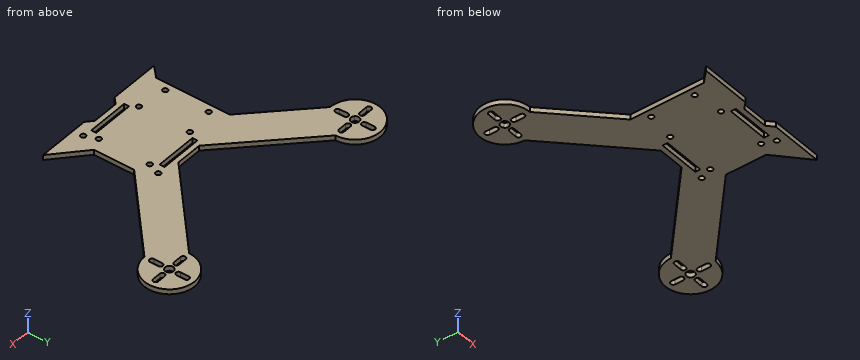
```python
from build123d import *

# Parameters (mm, degrees)
F0_R     = 1.5
F0_W     = 25
F0_H     = 3
F0_R_2   = 2.5
F1_DEPTH = 3


# Not quite as in the source:
# - ends of sketch curves that miss each other by under 0.0002 mm in the source are joined


with BuildPart() as f1:
    # F0 (on Top) → F1 (new body)
    with BuildSketch(Plane.XY):
        with BuildLine():
            Line((-10.0000000587, 25), (-55.7106781187, 70.7106779065))
            ThreePointArc((-55.7106781187, 70.7106779065), (-81.3172799026, 81.3172797703), (-70.7106779065, 55.7106781187))
            Line((-70.7106779065, 55.7106781187), (-37, 22.0000003253))
            Line((-37, 22.0000003253), (-37, -22.0000003253))
            Line((-37, -22.0000003253), (-43.4767450368, -28.4767453404))
            Line((-43.4767450368, -28.4767453404), (-13.4767454108, -28.4767453404))
            Line((-13.4767454108, -28.4767453404), (-10.0000000587, -25))
            Line((-10.0000000587, -25), (5.8262266936, -25))
            Line((5.8262266936, -25), (9.6204284269, -28.4767453404))
            Line((9.6204284269, -28.4767453404), (40.9900556349, -28.4767453404))
            Line((40.9900556349, -28.4767453404), (23, -11.9918965954))
            Line((23, -11.9918965954), (23, 11.9918965954))
            Line((23, 11.9918965954), (70.7106780935, 55.7106781187))
            ThreePointArc((70.7106780935, 55.7106781187), (81.3172798365, 81.3172798365), (55.7106781187, 70.7106779065))
            Line((55.7106781187, 70.7106779065), (5.8262266936, 25))
            Line((5.8262266936, 25), (-10.0000000587, 25))
        make_face()
        with Locations((-15.25, -15.25)):
            Circle(F0_R, mode=Mode.SUBTRACT)
        with Locations((-32.5, -13)):
            Circle(F0_R, mode=Mode.SUBTRACT)
        with Locations((-32.5, 13)):
            Circle(F0_R, mode=Mode.SUBTRACT)
        with Locations((-15.25, 15.25)):
            Circle(F0_R, mode=Mode.SUBTRACT)
        with Locations((18, -22.5)):
            Circle(F0_R, mode=Mode.SUBTRACT)
        with Locations((0, -20.5)):
            Rectangle(F0_W, F0_H, mode=Mode.SUBTRACT)
        with Locations((15.25, -15.25)):
            Circle(F0_R, mode=Mode.SUBTRACT)
        with Locations((0, 20.5)):
            Rectangle(F0_W, F0_H, mode=Mode.SUBTRACT)
        with Locations((15.25, 15.25)):
            Circle(F0_R, mode=Mode.SUBTRACT)
        with Locations((18, 22.5)):
            Circle(F0_R, mode=Mode.SUBTRACT)
        with BuildLine():
            ThreePointArc((-72.2106780183, 65.2703154499), (-70.7106780132, 66.7703154448), (-69.2106780183, 65.2703154398))
            Line((-69.2106780183, 65.2703154398), (-69.210678035, 60.2703154398))
            ThreePointArc((-69.210678035, 60.2703154398), (-70.7106780401, 58.7703154448), (-72.210678035, 60.2703154499))
            Line((-72.210678035, 60.2703154499), (-72.2106780183, 65.2703154499))
        make_face(mode=Mode.SUBTRACT)
        with BuildLine():
            ThreePointArc((-76.1510407975, 72.2106782191), (-74.6510407925, 70.7106782241), (-76.1510407874, 69.2106782191))
            Line((-76.1510407874, 69.2106782191), (-81.1510407874, 69.2106782023))
            ThreePointArc((-81.1510407874, 69.2106782023), (-82.6510407925, 70.7106781972), (-81.1510407975, 72.2106782023))
            Line((-81.1510407975, 72.2106782023), (-76.1510407975, 72.2106782191))
        make_face(mode=Mode.SUBTRACT)
        with BuildLine():
            ThreePointArc((-68.9429111657, 72.4784450716), (-68.4009792874, 71.6673866996), (-68.2106781187, 70.7106781187))
            ThreePointArc((-68.2106781187, 70.7106781187), (-69.7539695377, 68.4009792874), (-72.4784450716, 68.9429111657))
            ThreePointArc((-72.4784450716, 68.9429111657), (-72.4784450716, 72.4784450716), (-68.9429111657, 72.4784450716))
        make_face(mode=Mode.SUBTRACT)
        with BuildLine():
            Line((-60.2703154398, 69.210678035), (-65.2703154398, 69.2106780183))
            ThreePointArc((-65.2703154398, 69.2106780183), (-66.7703154448, 70.7106780132), (-65.2703154499, 72.2106780183))
            Line((-65.2703154499, 72.2106780183), (-60.2703154499, 72.210678035))
            ThreePointArc((-60.2703154499, 72.210678035), (-58.7703154448, 70.7106780401), (-60.2703154398, 69.210678035))
        make_face(mode=Mode.SUBTRACT)
        with BuildLine():
            Line((-69.210678, 81.1510407925), (-69.210678, 76.1510407925))
            ThreePointArc((-69.210678, 76.1510407925), (-70.710678, 74.6510407925), (-72.210678, 76.1510407925))
            Line((-72.210678, 76.1510407925), (-72.210678, 81.1510407925))
            ThreePointArc((-72.210678, 81.1510407925), (-70.710678, 82.6510407925), (-69.210678, 81.1510407925))
        make_face(mode=Mode.SUBTRACT)
        with BuildLine():
            ThreePointArc((65.2703154499, 72.2106780183), (66.7703154448, 70.7106780132), (65.2703154398, 69.2106780183))
            Line((65.2703154398, 69.2106780183), (60.2703154398, 69.210678035))
            ThreePointArc((60.2703154398, 69.210678035), (58.7703154448, 70.7106780401), (60.2703154499, 72.210678035))
            Line((60.2703154499, 72.210678035), (65.2703154499, 72.2106780183))
        make_face(mode=Mode.SUBTRACT)
        with BuildLine():
            Line((69.210678035, 60.2703154398), (69.2106780183, 65.2703154398))
            ThreePointArc((69.2106780183, 65.2703154398), (70.7106780132, 66.7703154448), (72.2106780183, 65.2703154499))
            Line((72.2106780183, 65.2703154499), (72.210678035, 60.2703154499))
            ThreePointArc((72.210678035, 60.2703154499), (70.7106780401, 58.7703154448), (69.210678035, 60.2703154398))
        make_face(mode=Mode.SUBTRACT)
        with Locations((70.7106781187, 70.7106781187)):
            Circle(F0_R_2, mode=Mode.SUBTRACT)
        with BuildLine():
            Line((81.1510407874, 69.2106782023), (76.1510407874, 69.2106782191))
            ThreePointArc((76.1510407874, 69.2106782191), (74.6510407925, 70.7106782241), (76.1510407975, 72.2106782191))
            Line((76.1510407975, 72.2106782191), (81.1510407975, 72.2106782023))
            ThreePointArc((81.1510407975, 72.2106782023), (82.6510407925, 70.7106781972), (81.1510407874, 69.2106782023))
        make_face(mode=Mode.SUBTRACT)
        with BuildLine():
            Line((72.210678, 81.1510407925), (72.210678, 76.1510407925))
            ThreePointArc((72.210678, 76.1510407925), (70.710678, 74.6510407925), (69.210678, 76.1510407925))
            Line((69.210678, 76.1510407925), (69.210678, 81.1510407925))
            ThreePointArc((69.210678, 81.1510407925), (70.710678, 82.6510407925), (72.210678, 81.1510407925))
        make_face(mode=Mode.SUBTRACT)
    extrude(amount=F1_DEPTH)


solid = f1.part
```
The listing builds one solid part. Answer for the finished solid, in the listing's coordinates (mm). Round coordinates to 2 decimals unless told otherwise and drop trailing zeros. Loops run counter-clockwise (first coordinate to the right, second up) from the corner with the lowest first, then second, coordinate; pieces in that order, holes last. Notation, with made-up numbers: (-15.75, 60.5) - (13.25, 60.5) arc R21 cw to (13.25, 76.5) - close; hole circle Ø8 at (-10, -16.75). An arc over 180 degrees is marked (long way). Return JSON: item names as keys, results as strings. Group by question number.
1. Consider probe 1 along Y at (x, z) = (3, 1.8); probe 2 along X at (y, z) = (-16, 1.3); probe 3 along X at (y, z) = (-16.5, 1.2). Determine where each line is inside the solid, lowest interval first.
2. The part is cut by section C-C on y = -6.5. Determine the outline of the cut face in (x, z).
3. The part is cut by section B-B on z = 0.85. State how many separate pieces and enclosed holes the cut face has, then the cut area to 3 significant figures.
4. The part is cut by section D-D on x = -52. Determine the outline of the cut face in (y, z), then the cut area to 3 significant figures.
5. The part is cut by section A-A on x = 7.5. Determine the outline of the cut face in (y, z).
6. Each of these flat-tipped pins is pushed along its axis until it touches: P1, Ø0.9, axis at y = 20, z = 1.5, coming from the -X side; P2, Ø1.5, axis at x = -1, z = 1.5, coming from the -Y side; P3, Ø0.9, axis at x = 63.5, z = 2, coming from the -Y side. Where does it stop, or does it pass through?
Resolved:
{
 "1": {"probe 1": "y = -25 to -22, -19 to 19, 22 to 25", "probe 2": "x = -37 to -16.55, -13.95 to 13.95, 16.55 to 27.37", "probe 3": "x = -37 to -16.08, -14.42 to 14.42, 16.08 to 27.92"},
 "2": {"outline": "(-37, 0) - (23, 0) - (23, 3) - (-37, 3) - close"},
 "3": {"separate pieces": "1", "enclosed holes": "20", "area": "6,610 mm²"},
 "4": {"outline": "(37, 0) - (67, 0) - (67, 3) - (37, 3) - close", "area": "90.0 mm²"},
 "5": {"outline": "(-26.53, 0) - (-22, 0) - (-22, 3) - (-26.53, 3) - close; (-19, 0) - (19, 0) - (19, 3) - (-19, 3) - close; (22, 0) - (26.53, 0) - (26.53, 3) - (22, 3) - close"},
 "6": {"P1": "stops at x = -37", "P2": "stops at y = -25", "P3": "stops at y = 48.69"}
}
